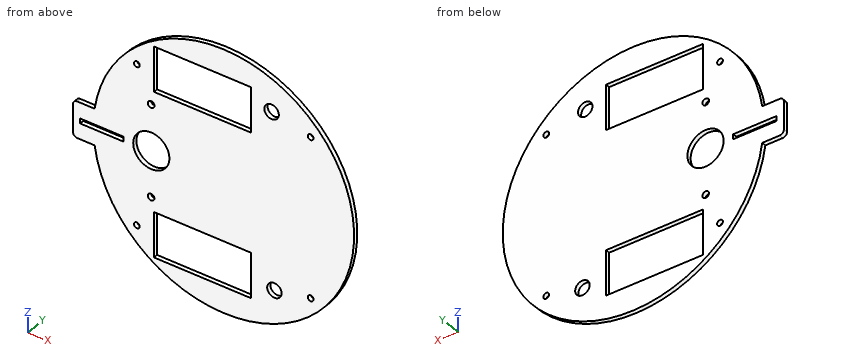
```python
from build123d import *

# Parameters (mm, degrees)
SKETCH_2_R          = 90
EXTRUDE_1_DEPTH     = 3
SKETCH_3_W          = 66.868711174
SKETCH_3_H          = 31
CUT_EXTRUDE_1_DEPTH = 3
SKETCH_4_R          = 12.5
CUT_EXTRUDE_2_DEPTH = 3
SKETCH_5_R          = 2
CUT_EXTRUDE_3_DEPTH = 3
SKETCH_6_R          = 5
CUT_EXTRUDE_4_DEPTH = 10
SKETCH_7_R          = 2.3
CUT_EXTRUDE_5_DEPTH = 3
EXTRUDE_2_DEPTH     = 3
SKETCH_9_W          = 30
SKETCH_9_H          = 3.4
CUT_EXTRUDE_6_DEPTH = 3


with BuildPart() as part:
    # 草圖2 → 填料-伸長1 (new body)
    with BuildSketch(Plane(origin=(0, 0, 0), x_dir=(1, 0, 0), z_dir=(0, 1, 0))):
        with Locations(Location((0, 0, 0), (0, 0, 270))):
            Circle(SKETCH_2_R)
    extrude(amount=EXTRUDE_1_DEPTH)

    # 草圖3 → 除料-伸長1 (cut)
    with BuildSketch(Plane(origin=(0, 3, 0), x_dir=(1, 0, 0), z_dir=(0, 1, 0))):
        with Locations((-14.765632174, 56.5)):
            Rectangle(SKETCH_3_W, SKETCH_3_H)
        with Locations((-14.765632174, -56.5)):
            Rectangle(SKETCH_3_W, SKETCH_3_H)
    extrude(amount=-CUT_EXTRUDE_1_DEPTH, mode=Mode.SUBTRACT)

    # 草圖4 → 除料-伸長2 (cut)
    with BuildSketch(Plane(origin=(0, 3, 0), x_dir=(1, 0, 0), z_dir=(0, 1, 0))):
        with Locations(Location((-50, 0, 0), (0, 0, 270))):
            Circle(SKETCH_4_R)
    extrude(amount=-CUT_EXTRUDE_2_DEPTH, mode=Mode.SUBTRACT)

    # 草圖5 → 除料-伸長3 (cut)
    with BuildSketch(Plane(origin=(0, 3, 0), x_dir=(1, 0, 0), z_dir=(0, 1, 0))):
        with Locations(Location((-60, 55, 0), (0, 0, 270))):
            Circle(SKETCH_5_R)
        with Locations(Location((-60, -55, 0), (0, 0, 270))):
            Circle(SKETCH_5_R)
        with Locations(Location((60, -55, 0), (0, 0, 270))):
            Circle(SKETCH_5_R)
        with Locations(Location((60, 55, 0), (0, 0, 270))):
            Circle(SKETCH_5_R)
    extrude(amount=-CUT_EXTRUDE_3_DEPTH, mode=Mode.SUBTRACT)

    # 草圖6 → 除料-伸長4 (cut)
    with BuildSketch(Plane(origin=(0, 3, 0), x_dir=(1, 0, 0), z_dir=(0, 1, 0))):
        with Locations(Location((35, 60, 0), (0, 0, 270))):
            Circle(SKETCH_6_R)
        with Locations(Location((33.043068023, -61.099555282, 0), (0, 0, 270))):
            Circle(SKETCH_6_R)
    extrude(amount=-CUT_EXTRUDE_4_DEPTH, mode=Mode.SUBTRACT)

    # 草圖7 → 除料-伸長5 (cut)
    with BuildSketch(Plane(origin=(0, 3, 0), x_dir=(1, 0, 0), z_dir=(0, 1, 0))):
        with Locations(Location((-50.137404534, -31.624669079, 0), (0, 0, 270))):
            Circle(SKETCH_7_R)
        with Locations(Location((-50.137404534, 31.624669079, 0), (0, 0, 270))):
            Circle(SKETCH_7_R)
    extrude(amount=-CUT_EXTRUDE_5_DEPTH, mode=Mode.SUBTRACT)

    # 草圖8 → 填料-伸長2 (add)
    with BuildSketch(Plane(origin=(0, 3, 0), x_dir=(1, 0, 0), z_dir=(0, 1, 0))):
        with BuildLine():
            Line((-89.12771735, 12.5), (-101.12771735, 12.5))
            ThreePointArc((-101.12771735, 12.5), (-103.249037693, 11.621320344), (-104.12771735, 9.5))
            Line((-104.12771735, 9.5), (-104.12771735, -9.5))
            ThreePointArc((-104.12771735, -9.5), (-103.249037693, -11.621320344), (-101.12771735, -12.5))
            Line((-101.12771735, -12.5), (-89.12771735, -12.5))
            Line((-89.12771735, -12.5), (-89.12771735, 12.5))
        make_face()
    extrude(amount=-EXTRUDE_2_DEPTH)

    # 草圖9 → 除料-伸長6 (cut)
    with BuildSketch(Plane(origin=(0, 3, 0), x_dir=(1, 0, 0), z_dir=(0, 1, 0))):
        with Locations((-84.12771735, 0)):
            Rectangle(SKETCH_9_W, SKETCH_9_H)
    extrude(amount=-CUT_EXTRUDE_6_DEPTH, mode=Mode.SUBTRACT)


solid = part.part
```
Can you work these out from the model? Positions are in its coordinate system, mm. Round coordinates to 2 decimals unless told otherwise and drop trailing zeros. Loops run counter-clockwise (first coordinate to the right, second up) from the corner with the lowest first, then second, coordinate; pieces in that order, holes last. Notation, with made-up numbers: (-13.75, 77) -> (17.25, 77) arc R22 ccw to (17.25, 87) -> close; hole circle Ø8 at (83.5, 59.25). An arc over 180 degrees is marked (long way). Answer in a Markdown table with one row per item.
Item 1: Suppose I cut it at A-A, the plane x = 0. List the corners of the cut face in (y, z) for me, plus the area to 3 significant figures.
Answer block:
| item | result |
|---|---|
| outline | (0, -90) -> (3, -90) -> (3, -72) -> (0, -72) -> close; (0, -41) -> (3, -41) -> (3, 41) -> (0, 41) -> close; (0, 72) -> (3, 72) -> (3, 90) -> (0, 90) -> close |
| area | 354 mm² |
Item 2: Suppose I cut it at D-D, the plane x = -78. List the corners of the cut face in (y, z) for me.
Answer block:
| item | result |
|---|---|
| outline | (0, -44.9) -> (3, -44.9) -> (3, -1.7) -> (0, -1.7) -> close; (0, 1.7) -> (3, 1.7) -> (3, 44.9) -> (0, 44.9) -> close |
Item 3: Suppose I cut it at C-C, the plane y = 1.8. Give the number of separate pieces and of enclosed holes in the cut face, plus the area to 3 significant figures.
Answer block:
| item | result |
|---|---|
| separate pieces | 1 |
| enclosed holes | 12 |
| area | 20,800 mm² |
Item 4: Suppose I cut it at B-B, the plane z = -60. List the corners of the cut face in (x, y) for me.
Answer block:
| item | result |
|---|---|
| outline | (-67.08, 0) -> (-48.2, 0) -> (-48.2, 3) -> (-67.08, 3) -> close; (18.67, 0) -> (30, 0) -> (30, 3) -> (18.67, 3) -> close; (40, 0) -> (67.08, 0) -> (67.08, 3) -> (40, 3) -> close |
Item 5: If I drill on probe 1 along X at (y, z) = (1.1, 0); probe 2 along X at (y, z) = (1.7, 59); probe 3 along Z at (x, y) = (-42.5, 2.45), over which ranges is the centre line in solid material (lowest first)?
Answer block:
| item | result |
|---|---|
| probe 1 | -104.13 to -99.13, -69.13 to -62.5, -37.5 to 90 |
| probe 2 | -67.96 to -48.2, 18.67 to 28.51, 37.58 to 67.96 |
| probe 3 | -79.33 to -72, -41 to -10, 10 to 41, 72 to 79.33 |
Item 6: Will these pins go through, and if not, where does the flat tip stop? P1, Ø1.5, axis at y = 1, z = -49.5, coming from the -X side; P2, Ø0.9, axis at x = -96.5, y = 1, coming from the +Z side; P3, Ø11.5, axis at x = 33.04, z = 61.1, coming from the +Y side; P4, Ø0.9, axis at y = 1, z = 55, coming from the +X side.
Answer block:
| item | result |
|---|---|
| P1 | x = -75.65 |
| P2 | z = 12.5 |
| P3 | y = 3 |
| P4 | x = 71.58 |
